Job drawing, mm, ordinate dimensions from the low corner. One solid piece. Give positions to 0.01 mm unless a question says otherwise; leave off trailing zeros. Order: outer loops, then holes, each group sorted by start corner. A loop starts at its lowest first (then second) coordinate and runs counter-clockwise, first axis right, second up.
Item 1: Band-saw the part on A-A on x = 1.7. Give the cut face in (y, z) (1 decimal), plus the area to 3 significant figures.
Item 2: Band-saw the part on B-B on z = 128. Give the cut face in (x, y).
Item 3: Wall check: L1, parallel to Y at x = 0.9, z = 78.5; L2, parallel to Z at x = 2.85, y = 30.5 (1 decimal); L3, parallel to Z at x = 1.65, y = 24.5. Give the ranges that are in metal, low to high.
Item 4: Band-saw the part on C-C on y = 23.5. Give the cut face in (x, z).
Item 5: Flat gauge pins, fed straight in: P1, Ø1.5, axis at x = 1, y = 37, coming from the +Z side (3 decimals); P2, Ø0.9, axis at x = 2, z = 164.5, coming from the -Y side; P3, Ø0.9, axis at x = 2, z = 141, coming from the +Y side. Where does each tip first touch, or does it go through?
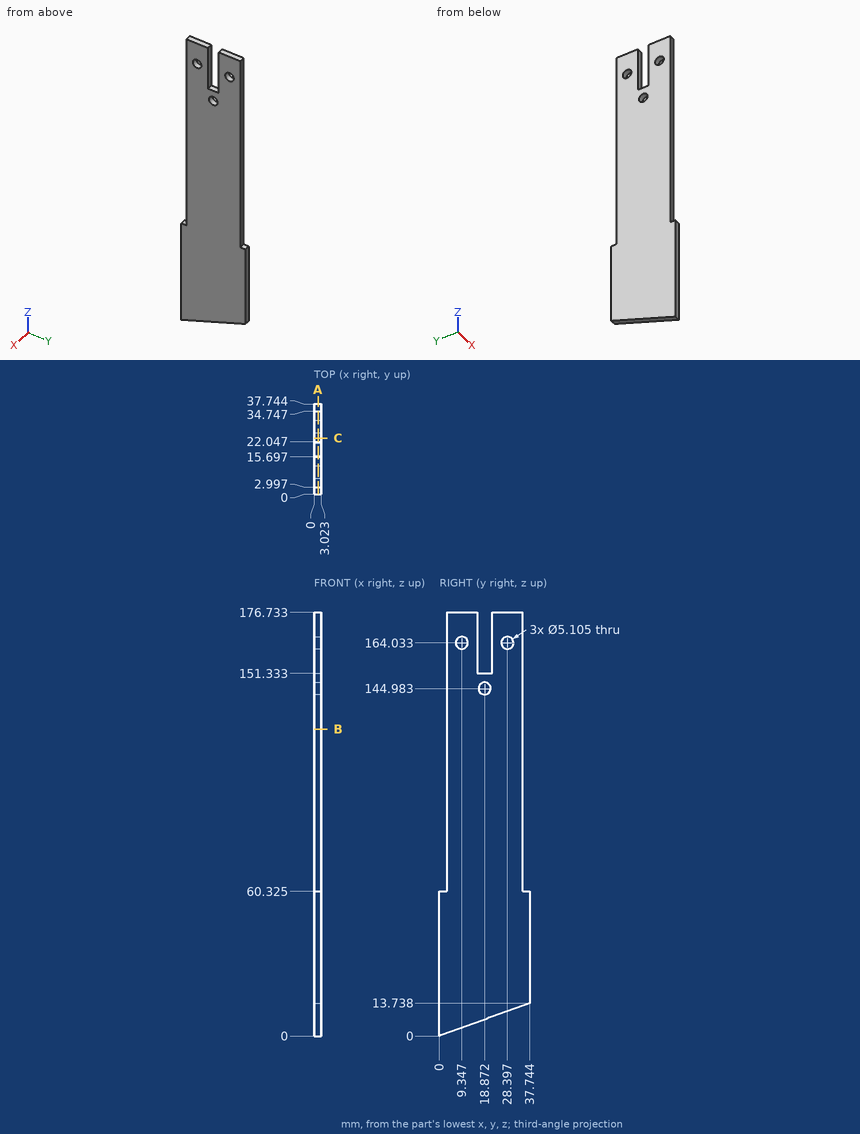
The answers:
1. outline: (0, 0) - (37.7, 13.7) - (37.7, 60.3) - (34.7, 60.3) - (34.7, 176.7) - (22, 176.7) - (22, 151.3) - (15.7, 151.3) - (15.7, 176.7) - (3, 176.7) - (3, 60.3) - (0, 60.3) - close; hole circle Ø5.1 at (9.3, 164); hole circle Ø5.1 at (18.9, 145); hole circle Ø5.1 at (28.4, 164)
1. area: 5,490 mm2
2. outline: (0, 3) - (3.02, 3) - (3.02, 34.75) - (0, 34.75) - close
3. L1: y = 3 to 34.75
3. L2: z = 11.1 to 162.6, 165.5 to 176.7
3. L3: z = 8.92 to 176.73
4. outline: (0, 8.55) - (3.02, 8.55) - (3.02, 176.73) - (0, 176.73) - close
5. P1: stops at z = 60.325
5. P2: stops at y = 3
5. P3: stops at y = 34.75
